The model under review builds one solid part; all positions refer to its coordinate system, in mm. Coordinates: 2 decimals unless noted, no trailing zeros. Loops run counter-clockwise (first coordinate to the right, second up) from the corner with the lowest first, then second, coordinate; pieces in that order, holes last. Notation, with made-up numbers: M 38,46.25 L 47,46.25 A31 cw 47,79.25 Z; hole C 43,-7 d2. An arc over 180 degrees is marked long. One line per item, written item: value.
```python
from build123d import *

# Parameters (mm, degrees)
F2_T = -5.08
F3_R = 0.508


with BuildPart() as f1:
    # F0 (on Front) → F1 (revolve)
    with BuildSketch(Plane.XZ):
        Polygon((0, 0), (0, 63.5), (-38.1, 63.5), (-26.903236725, 0), align=None)
    revolve(axis=Axis((0, 0, 31.75), (0, 0, 1)))

    # F2
    f2_openings = [f1.faces().sort_by_distance(p)[0] for p in [
        (0, 0, 63.5),
    ]]
    offset(amount=F2_T, openings=f2_openings)

    # F3
    f3_edges = [f1.edges().sort_by_distance(p)[0] for p in [
        (38.1, 0, 63.5),
        (32.941633, 0, 63.5),
    ]]
    fillet(f3_edges, radius=F3_R)


solid = f1.part
```
(1) Insertion check: pin 1 Ø12 at (x, y) = (9, -9) entering from -Z; pin 2 Ø1.5 at (x, z) = (6, 23.5) entering from -Y; pin 3 Ø6 at (x, z) = (5, 29.5) entering from +Y; pin 4 Ø12 at (x, z) = (-17, 33) entering from -Y. Each pin has a flat end and moves straight along its axis. Give the tip position at first contact, or say it passes through.
Checks:
pin 1: z = 0
pin 2: y = -30.66
pin 3: y = 32.37
pin 4: y = -31.09
(2) To check wall thickness, follow L1, parallel to Z at x = -5.5, y = 20.5; L2, parallel to Y at x = -6, z = 19; L3, parallel to Y at x = -4, z = 58. State the ranges of each line that lie inside material, in increasing order. Write a range as [from, to].
Checks:
L1: [0, 5.08]
L2: [-29.65, -24.37], [24.37, 29.65]
L3: [-36.91, -31.72], [31.72, 36.91]
(3) Add section A-A on x = 0. State the section outline as (y, z) points.
Checks:
outline: M -37.99,62.9 L -26.9,0 L 26.9,0 L 37.99,62.9 A0.51 ccw 37.49,63.5 L 33.37,63.5 A0.51 ccw 32.87,63.08 L 22.64,5.08 L -22.64,5.08 L -32.87,63.08 A0.51 ccw -33.37,63.5 L -37.49,63.5 A0.51 ccw Z
(4) Add section D-D on z = 7. State the section outline as (x, y) points, then the cut area to 3 significant figures.
Checks:
outline: C 0,0 d56.28; hole C 0,0 d45.96
area: 828 mm^2
(5) Add section C-C on z = 55. State the section outline as (x, y) points, then the cut area to 3 significant figures.
Checks:
outline: C 0,0 d73.2; hole C 0,0 d62.89
area: 1,100 mm^2
(6) Draft analysis for pull direction X (two halves, no side actions). For faces 1 (the face through (0, 0, 0)), 2 (the face through (5.8, 25.9, 27.2)), 3 (the face through (6.75, 30.4, 24.02)), 4 (the face through (0, 0, 5.08)), state which applies: pulls with the +X half, pulls with the -X half, needs draft (parallel to the pull), parting line crosses it, or undercut.
Checks:
face 1: needs draft
face 2: undercut
face 3: parting line crosses it
face 4: undercut
